Part model, mm, in its own coordinate system. A direction names the side the tool comes from. Give positions to 0.01 mm unless a question says otherwise; leave off trailing zeros. Loops run counter-clockwise (first coordinate to the right, second up) from the corner with the lowest first, then second, coordinate; pieces in that order, holes last. Notation, with made-up numbers: (65.5, -13) -> (81.5, -13) arc R25 cw to (81.5, 16) -> close; hole circle Ø4 at (26.25, 17). An arc over 180 degrees is marked (long way). Write item = value, one per line.
from build123d import *

# Parameters (mm, degrees)
F1_DEPTH = 25.4


# Not quite as in the source:
# - a feature of the source that left no trace in its solid (it failed there, or was rolled back) is left out


with BuildPart() as f1:
    # F0 (on Top) → F1 (new body)
    with BuildSketch(Plane.XY):
        with BuildLine():
            Line((0, 485.775), (0, 0))
            Line((0, 0), (63.5, 0))
            Line((63.5, 0), (63.5, 25.4))
            ThreePointArc((63.5, 25.4), (68.5094988016, 47.3970452561), (82.55, 65.0557372898))
            ThreePointArc((82.55, 65.0557372898), (96.5905011984, 82.7144293235), (101.6, 104.7114745797))
            Line((101.6, 104.7114745797), (101.6, 485.775))
            ThreePointArc((101.6, 485.775), (97.8802561211, 494.7552561211), (88.9, 498.475))
            Line((88.9, 498.475), (12.7, 498.475))
            ThreePointArc((12.7, 498.475), (3.7197438789, 494.7552561211), (0, 485.775))
        make_face()
    extrude(amount=F1_DEPTH)


solid = f1.part
1) Slice it at B-B, the plane y = 52. List the corners of the cut face in (x, z).
Resolved:
outline = (0, 0) -> (71.02, 0) -> (71.02, 25.4) -> (0, 25.4) -> close
2) Which spindle directions (+Z, -Z, +X, -X, +Y, -Y) get a long thin tool onto all of the face, cutting with end or side? Do faces 1 (the face through (63.5, 13, 13)), 2 (the face through (51, 498.475, 13)). Say none if no direction does.
Resolved:
face_1 = +Z, -Z, +X, -Y
face_2 = +Z, -Z, +X, -X, +Y
3) Drop flat-ended pins along their axis: P1, Ø3, axis at x = 30, y = 324.5, coming from the -Z side; P2, Ø7.5, axis at y = 12.5, z = 8.5, coming from the +X side; P3, Ø5, axis at x = 89.5, z = 21.5, coming from the -Y side. Give the stop position or say it passes through.
Resolved:
P1 = 0
P2 = 63.5
P3 = 69.07
4) Slice it at A-A, the plane z = 9.5. List the corners of the cut face in (x, y) (3 decimals).
Resolved:
outline = (0, 0) -> (63.5, 0) -> (63.5, 25.4) arc R50.8 cw to (82.55, 65.056) arc R50.8 ccw to (101.6, 104.711) -> (101.6, 485.775) arc R12.7 ccw to (88.9, 498.475) -> (12.7, 498.475) arc R12.7 ccw to (0, 485.775) -> close
5) Drill centre lines: line 1 along X through (y, z) = (37.5, 8); line 2 along Y through (x, z) = (94, 11.5); line 3 along Y through (x, z) = (7, 24.75). Where is each one in solid material? Low to high. Write a range as [from, to].
Resolved:
line_1 = [0, 64.96]
line_2 = [77.98, 497.41]
line_3 = [0, 497.12]
